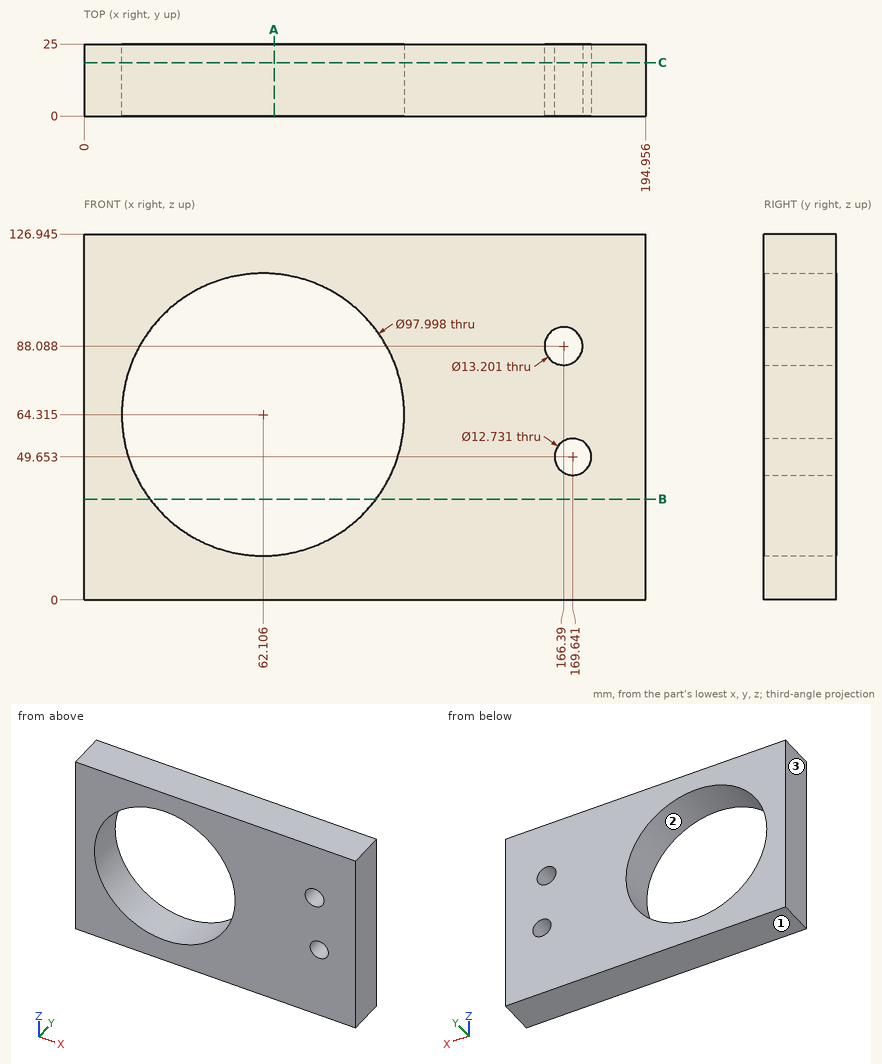
The figure shows three views and two pictorial views of one solid part (mm, origin at its lowest corner). Answer the questions. Give positions to 0.01 mm unless a question says otherwise; leave off trailing zeros. Order: outer loops, then holes, each group sorted by start corner. A loop starts at its lowest first (then second) coordinate and runs counter-clockwise, first axis right, second up. Notation, with made-up numbers: (53.5, 68.5) -> (57.5, 68.5) arc R34 cw to (57.5, 104.5) -> close; hole circle Ø6 at (36, 89). An arc over 180 degrees is marked (long way). Answer as CSV lines item,"result". Start each with the question number.
Q1. A cutting plane is placed at C-C (y = 18.5). Determine the outline of the cut face in (x, z) (1 decimal), then the cut area to 3 significant figures.
Q2. Given pin 1 (12 mm diameter, centred on y = 17, z = 38, fed in from -X), flat-ended and moving along its own axis, determine where the tip first touches the part or whether it passes through.
Q3. A cutting plane is placed at A-A (x = 66). Determine the outline of the cut face in (y, z) (1 decimal).
Q4. Find the intervals of material crossed by L1, parallel to X at y = 8, z = 83.5 (1 decimal); L2, parallel to Z at x = 63, y = 11 (1 decimal); L3, parallel to X at y = 4.5, z = 65.5 (1 decimal), in increasing order.
Q5. A cutting plane is placed at B-B (z = 35). Determine the outline of the cut face in (x, y), then the cut area to 3 significant figures.
Q6. Determine the mould class of the marked faces 1, 2 and 3 for opening direction X: pulls with the +X half, pulls with the -X half, needs draft (parallel to the pull), parting line crosses it, or undercut.
Results found:
1,outline,"(0, 0) -> (195, 0) -> (195, 126.9) -> (0, 126.9) -> close; hole circle Ø98 at (62.1, 64.3); hole circle Ø13.2 at (166.4, 88.1); hole circle Ø12.7 at (169.6, 49.7)"
1,area,"16,900 mm2"
2,pin 1,"x = 0"
3,outline,"(0, 0) -> (25, 0) -> (25, 15.5) -> (0, 15.5) -> close; (0, 113.2) -> (25, 113.2) -> (25, 126.9) -> (0, 126.9) -> close"
4,L1,"0 to 17, 107.2 to 161.6, 171.1 to 195"
4,L2,"0 to 15.3, 113.3 to 126.9"
4,L3,"0 to 13.1, 111.1 to 195"
5,outline,"(0, 0) -> (22.84, 0) -> (22.84, 25) -> (0, 25) -> close; (101.37, 0) -> (194.96, 0) -> (194.96, 25) -> (101.37, 25) -> close"
5,area,"2,910 mm2"
6,face 1,"needs draft"
6,face 2,"undercut"
6,face 3,"pulls with the -X half"
